Part model, mm, in its own coordinate system. Round coordinates to 2 decimals unless told otherwise and drop trailing zeros. Order: outer loops, then holes, each group sorted by start corner. A loop starts at its lowest first (then second) coordinate and runs counter-clockwise, first axis right, second up. Notation, with made-up numbers: (-16.75, 40.25) -> (6.25, 40.25) arc R21 cw to (6.25, 54.25) -> close; hole circle Ø7 at (-33, -9.75). An arc over 180 degrees is marked (long way). Return JSON: item names as keys, results as strings. Group by question number.
from build123d import *

# Parameters (mm, degrees)
SKETCH_1_R      = 35
SKETCH_1_R_2    = 1.5
EXTRUDE_1_DEPTH = 1


with BuildPart() as part:
    # Sketch 1 → Extrude 1 (new body)
    with BuildSketch(Plane(origin=(0, 0, 0), x_dir=(1, 0, 0), z_dir=(0, 1, 0))):
        with Locations(Location((0, 0, 0), (0, 0, 270))):
            Circle(SKETCH_1_R)
        with BuildLine():
            Line((-20.493901532, -16), (20.493901532, -16))
            ThreePointArc((20.493901532, -16), (0, -26), (-20.493901532, -16))
        make_face(mode=Mode.SUBTRACT)
        with BuildLine():
            Line((-18, -10), (-24, -10))
            ThreePointArc((-24, -10), (-26, 0), (-24, 10))
            Line((-24, 10), (-18, 10))
            Line((-18, 10), (24, 10))
            ThreePointArc((24, 10), (26, 0), (24, -10))
            Line((24, -10), (-18, -10))
        make_face(mode=Mode.SUBTRACT)
        with Locations(Location((-18, -13, 0), (0, 0, 270))):
            Circle(SKETCH_1_R_2, mode=Mode.SUBTRACT)
        with Locations(Location((-9, -13, 0), (0, 0, 270))):
            Circle(SKETCH_1_R_2, mode=Mode.SUBTRACT)
        with Locations(Location((0, -13, 0), (0, 0, 270))):
            Circle(SKETCH_1_R_2, mode=Mode.SUBTRACT)
        with Locations(Location((9, -13, 0), (0, 0, 270))):
            Circle(SKETCH_1_R_2, mode=Mode.SUBTRACT)
        with Locations(Location((18, -13, 0), (0, 0, 270))):
            Circle(SKETCH_1_R_2, mode=Mode.SUBTRACT)
        with Locations(Location((-21.566756826, -21.566756826, 0), (0, 0, 270))):
            Circle(SKETCH_1_R_2, mode=Mode.SUBTRACT)
        with Locations(Location((-30.5, 0, 0), (0, 0, 270))):
            Circle(SKETCH_1_R_2, mode=Mode.SUBTRACT)
        with Locations(Location((0, -30.5, 0), (0, 0, 270))):
            Circle(SKETCH_1_R_2, mode=Mode.SUBTRACT)
        with Locations(Location((21.566756826, -21.566756826, 0), (0, 0, 270))):
            Circle(SKETCH_1_R_2, mode=Mode.SUBTRACT)
        with Locations(Location((-21.566756826, 21.566756826, 0), (0, 0, 270))):
            Circle(SKETCH_1_R_2, mode=Mode.SUBTRACT)
        with BuildLine():
            ThreePointArc((-20.493901532, 16), (0, 26), (20.493901532, 16))
            Line((20.493901532, 16), (-20.493901532, 16))
        make_face(mode=Mode.SUBTRACT)
        with Locations(Location((0, 30.5, 0), (0, 0, 270))):
            Circle(SKETCH_1_R_2, mode=Mode.SUBTRACT)
        with Locations(Location((21.566756826, 21.566756826, 0), (0, 0, 270))):
            Circle(SKETCH_1_R_2, mode=Mode.SUBTRACT)
        with Locations(Location((30.5, 0, 0), (0, 0, 270))):
            Circle(SKETCH_1_R_2, mode=Mode.SUBTRACT)
        with Locations(Location((18, 13, 0), (0, 0, 270))):
            Circle(SKETCH_1_R_2, mode=Mode.SUBTRACT)
        with Locations(Location((-18, 13, 0), (0, 0, 270))):
            Circle(SKETCH_1_R_2, mode=Mode.SUBTRACT)
        with Locations(Location((-9, 13, 0), (0, 0, 270))):
            Circle(SKETCH_1_R_2, mode=Mode.SUBTRACT)
        with Locations(Location((0, 13, 0), (0, 0, 270))):
            Circle(SKETCH_1_R_2, mode=Mode.SUBTRACT)
        with Locations(Location((9, 13, 0), (0, 0, 270))):
            Circle(SKETCH_1_R_2, mode=Mode.SUBTRACT)
    extrude(amount=EXTRUDE_1_DEPTH)


solid = part.part
(1) Saw through at D-D, the plane z = -13. List the corners of the cut face in (x, y).
(2) Saw through at A-A, the plane z = 0. List the corners of the cut face in (x, y), and give its area (3 significant figures).
(3) Saw through at B-B, the plane x = 18. List the corners of the cut face in (y, z).
(4) Saw through at C-C, the plane x = -30.5. List the corners of the cut face in (y, z), and give its area (3 significant figures).
(5) Mould opens along Z. For faces 1 (the cylindrical face through (-21.3, 0.49, -27.77)), 2 (the flat face through (3, 1, -11)), 3 (the cylindrical face through (-9.9, 0.5, -14.2)) say: pulls with the +Z half, pulls with the -Z half, needs draft (parallel to the pull), parting line crosses it, or undercut.
(6) Probe L1, parallel to Z at x = 13, y = 0.7; L2, parallel to X at y = 0.3, z = 13; L3, parallel to X at y = 0.65, z = 0. List the from-to ranges inside material, lowest first. Write a range as [from, to].
(7) Pin check, flat tips, straight feed: P1, Ø2.5, axis at x = 9, z = 13, coming from the +Y side; P2, Ø0.5, axis at x = 7, y = 0.5, coming from the -Z side. Stop position of each tip, or through.
Results are:
{
 "1": {"outline": "(-32.5, 0) -> (-19.5, 0) -> (-19.5, 1) -> (-32.5, 1) -> close; (-16.5, 0) -> (-10.5, 0) -> (-10.5, 1) -> (-16.5, 1) -> close; (-7.5, 0) -> (-1.5, 0) -> (-1.5, 1) -> (-7.5, 1) -> close; (1.5, 0) -> (7.5, 0) -> (7.5, 1) -> (1.5, 1) -> close; (10.5, 0) -> (16.5, 0) -> (16.5, 1) -> (10.5, 1) -> close; (19.5, 0) -> (32.5, 0) -> (32.5, 1) -> (19.5, 1) -> close"},
 "2": {"outline": "(-35, 0) -> (-32, 0) -> (-32, 1) -> (-35, 1) -> close; (-29, 0) -> (-26, 0) -> (-26, 1) -> (-29, 1) -> close; (26, 0) -> (29, 0) -> (29, 1) -> (26, 1) -> close; (32, 0) -> (35, 0) -> (35, 1) -> (32, 1) -> close", "area": "12.0 mm^2"},
 "3": {"outline": "(0, -30.02) -> (1, -30.02) -> (1, -18.76) -> (0, -18.76) -> close; (0, -16) -> (1, -16) -> (1, -14.5) -> (0, -14.5) -> close; (0, -11.5) -> (1, -11.5) -> (1, -10) -> (0, -10) -> close; (0, 10) -> (1, 10) -> (1, 11.5) -> (0, 11.5) -> close; (0, 14.5) -> (1, 14.5) -> (1, 16) -> (0, 16) -> close; (0, 18.76) -> (1, 18.76) -> (1, 30.02) -> (0, 30.02) -> close"},
 "4": {"outline": "(0, -17.17) -> (1, -17.17) -> (1, -1.5) -> (0, -1.5) -> close; (0, 1.5) -> (1, 1.5) -> (1, 17.17) -> (0, 17.17) -> close", "area": "31.3 mm^2"},
 "5": {"face 1": "parting line crosses it", "face 2": "needs draft", "face 3": "undercut"},
 "6": {"L1": "z = [-32.5, -22.52], [-16, -10], [10, 16], [22.52, 32.5]", "L2": "x = [-32.5, -19.5], [-16.5, -10.5], [-7.5, -1.5], [1.5, 7.5], [10.5, 16.5], [19.5, 32.5]", "L3": "x = [-35, -32], [-29, -26], [26, 29], [32, 35]"},
 "7": {"P1": "passes through", "P2": "stops at z = -34.34"}
}
